Autodesk Inventor part; units mm, degrees
ref_plane "YZ Plane" through (0, 0, 0) normal (1, 0, 0) x (0, 1, 0)
ref_plane "XZ Plane" through (0, 0, 0) normal (0, 1, 0) x (-1, 0, 0)
ref_plane "XY Plane" through (0, 0, 0) normal (0, 0, 1) x (1, 0, 0)
sketch "Sketch1" plane through (0, 0, 0) normal (0, 1, 0) x (-1, 0, 0)
  line L0 (-10.16, 10.16) -> (10.16, 10.16)
  line L1 (10.16, 10.16) -> (10.16, -10.16)
  line L2 (10.16, -10.16) -> (-10.16, -10.16)
  line L3 (-10.16, -10.16) -> (-10.16, 10.16)
  circle A0 centre (0, 0) radius 8.255
  dimension "d0" = 20.32
  dimension "d1" = 20.32
  dimension "d2" = 10.16
  dimension "d3" = 10.16
  dimension "d4" = 16.51
extrude "Extrusion1" add sketch "Sketch1" along normal blind 12.7
sketch "Sketch2" plane through (10.16, 0, 10.16) normal (1, 0, 0) x (0, 0, -1)
  line L0 (1.778, 12.446) -> (2.921, 5.08)
  line L1 (2.921, 5.08) -> (17.399, 5.08)
  line L2 (17.399, 5.08) -> (18.542, 12.446)
  line L3 (18.542, 12.446) -> (1.778, 12.446)
  line L4 (20.32, 0) -> (0, 0)
  line L5 (20.32, 0) -> (20.32, 12.7)
  point P0 (10.16, 0)
  dimension "d7" = 16.764
  dimension "d8" = 14.478
  dimension "d9" = 7.366
  dimension "d10" = 5.08
  dimension "d11" = 2.921
extrude "Extrusion2" add sketch "Sketch2" along normal blind 12.7
sketch "Sketch3" plane through (10.16, 12.446, 8.382) normal (0, 1, 0) x (1, 0, 0)
  circle A0 centre (5.842, 8.382) radius 2.286
  line L0 (12.7, 16.764) -> (12.7, 0)
  point P0 (-10.16, 8.382)
  dimension "d14" = 4.572
  dimension "d15" = 6.858
extrude "Extrusion3" cut sketch "Sketch3" against normal blind 17.78
sketch "Sketch4" plane through (10.16, 12.446, 8.382) normal (0, 1, 0) x (1, 0, 0)
  circle A0 centre (5.842, 8.382) radius 2.286
  line L0 (0, 0) -> (0, 16.764)
  line L1 (0, 0) -> (12.7, 0)
  line L2 (12.7, 16.764) -> (12.7, 0)
  line L3 (0, 16.764) -> (12.7, 16.764)
  point P0 (-10.16, 8.382)
extrude "Extrusion4" add sketch "Sketch4" along normal up to surface (0.254 mm away)
sketch "Sketch5" plane through (0, 0, 0) normal (0, -1, 0) x (1, 0, 0)
  line L0 (14.2823, 20.4865) -> (-14.5737, 20.4865)
  line L1 (-14.5737, 20.4865) -> (-14.5737, -26.9822)
  line L2 (-14.5737, -26.9822) -> (14.2823, -26.9822)
  line L3 (14.2823, -26.9822) -> (14.2823, 20.4865)
  point P0 (0, 0)
extrude "Extrusion5" cut sketch "Sketch5" against normal blind 2.54
properties part number "HopperFinal3"
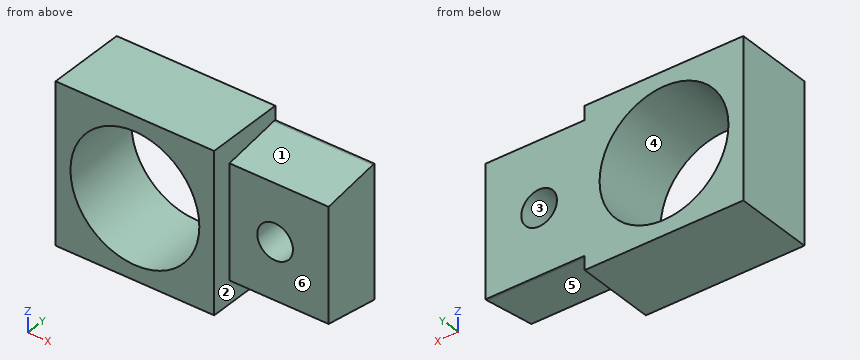
Work out the finished part from the listing and answer in its coordinate system (mm). Face numbers are marked on the shaded views. A direction names the side the tool comes from. Round coordinates to 2 decimals unless told otherwise and drop trailing zeros. Write each loop counter-clockwise with the first axis right and the second up, starting at its lowest first coordinate (ties: lowest second). Pieces come first, ordered by that corner, then holes. Notation, with made-up numbers: (22.25, 23) - (40.25, 23) arc R32 ccw to (40.25, 51) - close; hole circle Ø4 at (88, -3.75). An arc over 180 degrees is marked (long way). Answer in a Markdown table with one row per item. Add a question column.
1. Given pin 1 (6.5 mm diameter, centred on x = 14, z = -0.5, fed in from -Y), flat-ended and moving along its own axis, determine where the tip first touches the part or whether it passes through.
2. For the marked faces 4, 5 and 6, determine the directions among +Z, -Z, +X, -X, +Y, -Y from which every point of the face is accessible in a straight line to the end or side of a thin tool.
3. A cutting plane is placed at D-D, the plane z = -3. Determine the outline of the cut face in (x, y).
4. Find the intervals of material crossed by line 1 along X through (y, z) = (7.25, 0) (3 decimals); line 2 along X through (y, z) = (10.25, -2); line 3 along X through (y, z) = (5, 0.25), in increasing order. Write a range as from..to.
5. The mould has two halves that part along Z. Classify the marked faces 1, 2 and 3: +Z half, -Z half, draft (parallel to the pull), parting line (faces both ways), or undercut.
6. A cutting plane is placed at A-A, the plane x = 0. Determine the outline of the cut face in (y, z) (3 decimals), and give its area (3 significant figures).
7. A cutting plane is placed at C-C, the plane y = 8. Determine the outline of the cut face in (x, z) (3 decimals).
8. A cutting plane is placed at B-B, the plane z = 0. Determine the outline of the cut face in (x, y) (3 decimals).
Worked out:
| question | item | result |
|---|---|---|
| 1 | pin 1 | y = 5.08 |
| 2 | face 4 | +Y, -Y |
| 2 | face 5 | -Z, +X, -Y |
| 2 | face 6 | +Z, -Z, +X, -Y |
| 3 | outline | (-10.16, 2.54) - (-7.69, 2.54) - (-7.69, 12.7) - (-10.16, 12.7) - close; (7.69, 2.54) - (10.16, 2.54) - (10.16, 5.08) - (22.86, 5.08) - (22.86, 12.7) - (7.69, 12.7) - close |
| 4 | line 1 | -10.16..-8.255, 8.255..13.716, 18.288..22.86 |
| 4 | line 2 | -10.16..-8.01, 8.01..14.89, 17.11..22.86 |
| 4 | line 3 | -10.16..-8.25, 8.25..10.16 |
| 5 | face 1 | +Z half |
| 5 | face 2 | draft |
| 5 | face 3 | undercut |
| 6 | outline | (2.54, -10.16) - (12.7, -10.16) - (12.7, -8.255) - (2.54, -8.255) - close; (2.54, 8.255) - (12.7, 8.255) - (12.7, 10.16) - (2.54, 10.16) - close |
| 6 | area | 38.7 mm^2 |
| 7 | outline | (-10.16, -10.16) - (10.16, -10.16) - (10.16, -7.692) - (22.86, -7.692) - (22.86, 7.692) - (10.16, 7.692) - (10.16, 10.16) - (-10.16, 10.16) - close; hole circle Ø16.51 at (0, 0); hole circle Ø4.572 at (16.002, 0) |
| 8 | outline | (-10.16, 2.54) - (-8.255, 2.54) - (-8.255, 12.7) - (-10.16, 12.7) - close; (8.255, 2.54) - (10.16, 2.54) - (10.16, 5.08) - (13.716, 5.08) - (13.716, 12.7) - (8.255, 12.7) - close; (18.288, 5.08) - (22.86, 5.08) - (22.86, 12.7) - (18.288, 12.7) - close |
